Here's how the part is built. I have some questions about the finished solid (model axes, mm). A direction names the side the tool comes from. Coordinates: 2 decimals unless noted, no trailing zeros. Write each loop counter-clockwise with the first axis right and the second up, starting at its lowest first coordinate (ties: lowest second). Pieces come first, ordered by that corner, then holes.
```python
from build123d import *

# Parameters (mm, degrees)
CROQUIS1_W              = 55
CROQUIS1_H              = 55
CROQUIS1_R              = 1.5
SALIENTE_EXTRUIR1_DEPTH = 2
CROQUIS3_W              = 65
CROQUIS3_H              = 65
CROQUIS3_W_2            = 55
CROQUIS3_H_2            = 55
SALIENTE_EXTRUIR2_DEPTH = 2
CROQUIS4_R              = 2.7
CORTAR_EXTRUIR1_DEPTH   = 2


with BuildPart() as part:
    # Croquis1 → Saliente-Extruir1 (new body)
    with BuildSketch(Plane(origin=(0, 0, 0), x_dir=(1, 0, 0), z_dir=(0, 1, 0))):
        with Locations((27.5, 27.5)):
            Rectangle(CROQUIS1_W, CROQUIS1_H)
        with Locations(Location((1.75, 42.5, 0), (0, 0, 270))):
            Circle(CROQUIS1_R, mode=Mode.SUBTRACT)
        with Locations(Location((1.75, 12.5, 0), (0, 0, 270))):
            Circle(CROQUIS1_R, mode=Mode.SUBTRACT)
        with Locations(Location((53.25, 42.5, 0), (0, 0, 90))):
            Circle(CROQUIS1_R, mode=Mode.SUBTRACT)
        with Locations(Location((53.25, 12.5, 0), (0, 0, 90))):
            Circle(CROQUIS1_R, mode=Mode.SUBTRACT)
        Polygon((13.5, 13.5), (27.5, 13.5), (41.5, 13.5), (41.5, 28.15), (41.5, 41.5), (27.5, 41.5), (13.5, 41.5), (13.5, 27.5), align=None, mode=Mode.SUBTRACT)
    extrude(amount=SALIENTE_EXTRUIR1_DEPTH)

    # Croquis3 → Saliente-Extruir2 (add)
    with BuildSketch(Plane(origin=(0, 2, 0), x_dir=(1, 0, 0), z_dir=(0, 1, 0))):
        with Locations((27.5, 27.5)):
            Rectangle(CROQUIS3_W, CROQUIS3_H)
        with Locations((27.5, 27.5)):
            Rectangle(CROQUIS3_W_2, CROQUIS3_H_2, mode=Mode.SUBTRACT)
    extrude(amount=-SALIENTE_EXTRUIR2_DEPTH)

    # Croquis4 → Cortar-Extruir1 (cut)
    with BuildSketch(Plane(origin=(0, 2, 0), x_dir=(1, 0, 0), z_dir=(0, 1, 0))):
        with Locations(Location((53.25, 42.5, 0), (0, 0, 270))):
            Circle(CROQUIS4_R)
        with Locations(Location((53.25, 12.5, 0), (0, 0, 270))):
            Circle(CROQUIS4_R)
        with Locations(Location((1.75, 12.5, 0), (0, 0, 270))):
            Circle(CROQUIS4_R)
        with Locations(Location((1.75, 42.5, 0), (0, 0, 270))):
            Circle(CROQUIS4_R)
    extrude(amount=-CORTAR_EXTRUIR1_DEPTH, mode=Mode.SUBTRACT)


solid = part.part
```
1) Will this pin go through, and if not, where does the flat tip stop? pin 1 (4.5 mm diameter, centred on x = 1.75, z = -12.5, fed in from +Y).
Values follow:
pin 1: passes through
2) On a 3-axis mill with a long thin cutter (end or side, diameter ignored), from which of +Z, -Z, +X, -X, +Y, -Y can I reach the whole of each face in a straight line? I mean faces 1 (the face through (27, 1, -41.5)), 2 (the face through (-5, 1, -27)). Say none if no direction works.
Values follow:
face 1: +Y, -Y
face 2: +Z, -Z, -X, +Y, -Y
3) Imagine slicing it at D-D on x = 40.5. Please give me the cut outline in (y, z).
Values follow:
outline: (0, -60) - (2, -60) - (2, -41.5) - (0, -41.5) - close; (0, -13.5) - (2, -13.5) - (2, 5) - (0, 5) - close
4) Imagine slicing it at B-B on z = -12.5. Please give me the cut outline in (x, y).
Values follow:
outline: (-5, 0) - (-0.95, 0) - (-0.95, 2) - (-5, 2) - close; (4.45, 0) - (50.55, 0) - (50.55, 2) - (4.45, 2) - close; (55.95, 0) - (60, 0) - (60, 2) - (55.95, 2) - close
5) Imagine slicing it at A-A on x = 53.25. Please give me the cut outline in (y, z).
Values follow:
outline: (0, -60) - (2, -60) - (2, -45.2) - (0, -45.2) - close; (0, -39.8) - (2, -39.8) - (2, -15.2) - (0, -15.2) - close; (0, -9.8) - (2, -9.8) - (2, 5) - (0, 5) - close
6) I need wall thicknesses on probe 1 along X at (y, z) = (0.95, -42.5); probe 2 along Z at (x, y) = (53.5, 1.4); probe 3 along Z at (x, y) = (20.5, 1.5). Which ranges of each line are inside material? Lowest first, please.
Values follow:
probe 1: x = -5 to -0.95, 4.45 to 50.55, 55.95 to 60
probe 2: z = -60 to -45.19, -39.81 to -15.19, -9.81 to 5
probe 3: z = -60 to -41.5, -13.5 to 5
7) Imagine slicing it at C-C on y = 1.3. Please give me the cut outline in (x, z).
Values follow:
outline: (-5, -60) - (60, -60) - (60, 5) - (-5, 5) - close; hole circle Ø5.4 at (1.75, -42.5); hole circle Ø5.4 at (1.75, -12.5); hole (13.5, -41.5) - (41.5, -41.5) - (41.5, -13.5) - (13.5, -13.5) - close; hole circle Ø5.4 at (53.25, -42.5); hole circle Ø5.4 at (53.25, -12.5)
8) We'd pull the mould along Z, two halves only. Please class faces 3 (the face through (13, 0, -28)), 4 (the face through (27, 1, -60)), 5 (the face through (27, 1, 5)), 6 (the face through (41.5, 1, -28)): pulls with the +Z half, pulls with the -Z half, needs draft (parallel to the pull), parting line crosses it, or undercut.
Values follow:
face 3: needs draft
face 4: pulls with the -Z half
face 5: pulls with the +Z half
face 6: undercut
